Build history of the part. All positions in model axes, mm. A direction names the side the tool comes from. Give positions to 0.01 mm unless a question says otherwise; leave off trailing zeros. Order: outer loops, then holes, each group sorted by start corner. A loop starts at its lowest first (then second) coordinate and runs counter-clockwise, first axis right, second up. Notation, with made-up numbers: (67, 36) - (108, 36) arc R27 cw to (108, 75) - close; hole circle Ø7 at (-33, 69). An arc over 180 degrees is marked (long way). Use a Markdown table: item, result.
from build123d import *

# Parameters (mm, degrees)
F0_R     = 4
F1_DEPTH = 5
F0_R_2   = 11
F0_R_3   = 5.5
F2_DEPTH = 3.5
F5_DEPTH = 1.5


with BuildPart() as f1:
    # F0 (on Top) → F1 (new body)
    with BuildSketch(Plane.XY):
        Circle(F0_R)
    extrude(amount=F1_DEPTH)

    # F0 (on Top) → F2 (join)
    with BuildSketch(Plane.XY):
        Circle(F0_R_2)
        Circle(F0_R_3, mode=Mode.SUBTRACT)
        Circle(F0_R_3)
        Circle(F0_R, mode=Mode.SUBTRACT)
        Circle(F0_R)
    extrude(amount=-F2_DEPTH)

    # F3 (on Right) → F4 (revolve, cut)
    with BuildSketch(Plane.YZ):
        with BuildLine():
            Line((0, -33.02), (0, -2.286))
            ThreePointArc((0, -2.286), (-30.734, -33.02), (0, -63.754))
            Line((0, -63.754), (0, -33.02))
        make_face()
    revolve(axis=Axis((0, 0, -16.51), (0, 0, 1)), mode=Mode.SUBTRACT)

    # F0 (on Top) → F5 (join)
    with BuildSketch(Plane.XY):
        Circle(F0_R_3)
        Circle(F0_R, mode=Mode.SUBTRACT)
    extrude(amount=F5_DEPTH)


solid = f1.part
1) Slice it at A-A (x = 0). Write the cut outline in (y, z).
Computed:
| item | result |
|---|---|
| outline | (-11, -3.5) - (-8.55, -3.5) arc R30.73 cw to (8.55, -3.5) - (11, -3.5) - (11, 0) - (5.5, 0) - (5.5, 1.5) - (4, 1.5) - (4, 5) - (-4, 5) - (-4, 1.5) - (-5.5, 1.5) - (-5.5, 0) - (-11, 0) - close |
2) Slice it at D-D (z = 3.5). Write the cut outline in (x, y), and give its area (3 significant figures).
Computed:
| item | result |
|---|---|
| outline | circle Ø8 at (0, 0) |
| area | 50.3 mm² |
3) Pin check, flat tips, straight feed: P1, Ø1, axis at y = 6.5, z = -2, coming from the -X side; P2, Ø3, axis at y = 2, z = 3.5, coming from the +X side; P3, Ø3, axis at y = -4, z = 2.5, coming from the +X side. Stop position of each tip, or through.
Computed:
| item | result |
|---|---|
| P1 | stops at x = -9.22 |
| P2 | stops at x = 3.97 |
| P3 | stops at x = 4.68 |
4) Slice it at C-C (z = -2). Write the cut outline in (x, y), and give its area (3 significant figures).
Computed:
| item | result |
|---|---|
| outline | circle Ø22 at (0, 0) |
| area | 380 mm² |
5) Tool access for faces 1 (the flat face through (-3, 5, 0)), 2 (the flat face through (0, 0, 5)): list every direction of +Z, -Z, +X, -X, +Y, -Y with a clear straight run to the whole face (end or side of a thin tool).
Computed:
| item | result |
|---|---|
| face 1 | +Z |
| face 2 | +Z, +X, -X, +Y, -Y |
6) Wall check: line 1 (Z direction, x = 8.5, y = 6.75); line 2 (X direction, y = 9.75, z = -3); line 3 (X direction, y = 8, z = -0.25). Give the ranges that are in metal, low to high. Write a range as from..to.
Computed:
| item | result |
|---|---|
| line 1 | z = -3.5..0 |
| line 2 | x = -5.09..5.09 |
| line 3 | x = -7.55..7.55 |
